Here's how the part is built. I have some questions about the finished solid (model axes, mm). A direction names the side the tool comes from. Round coordinates to 2 decimals unless told otherwise and drop trailing zeros. Loops run counter-clockwise (first coordinate to the right, second up) from the corner with the lowest first, then second, coordinate; pieces in that order, holes last. Notation, with made-up numbers: (52.5, 60) -> (57.5, 60) arc R16 cw to (57.5, 87) -> close; hole circle Ø6 at (-32.75, -33.5). An arc over 180 degrees is marked (long way). Use one line per item in the form item = value. Start each with the question number.
Item 1: Thinking about a two-plate mould opening in Z: for faces 1 (the face through (0.15, 207.27, 2.14)), 2 (the face through (-2, 156, 6)), 3 (the face through (2, 119, 4.3)), which applies, released by +Z, released by -Z, zero draft, split by the parting line, or undercut?
Item 2: If we section it at A-A (y = 172): Write out the boundary of the cut face in (x, z) (3 decimals).
Item 3: For faces 4 (the face through (-1.57, 205.91, 3.09)), 5 (the face through (-2, 21, 6)), 6 (the face through (-3, 238, 4)), which set-ups out of +Z, -Z, +X, -X, +Y, -Y let a thin tool reach every point of the face, with its end or its side?
Item 4: I'm going to push flat-ended pins straight in: pin 1 Ø3 at (y, z) = (20, 4.914) entering from -X; pin 2 Ø4 at (y, z) = (20.5, 4) entering from -X; pin 3 Ø0.6 at (x, y) = (1, 31) entering from +Z; pin 4 Ø2 at (y, z) = (85, 4.914) entering from +X. Where does each tip first touch, or does it pass through?
Item 5: If I drill on L1, parallel to Z at x = -1.25, y = 20; L2, parallel to Y at x = -4.25, z = 3.5; L3, parallel to Y at x = 1, z = 2, over which ranges is the centre line in solid material (lowest first)? Write a range as [from, to].
Autodesk Fusion 360 part; units mm, degrees
sketch "Skizze1" plane through (0, 0, 0) normal (0, 1, 0) x (1, 0, 0)
  line L0 (-29.0267, 0) -> (32.308, 0) construction
  line L1 (0, -25.3668) -> (0, 26.124) construction
  line L2 (0, 0) -> (0, -10)
  line L3 (0, -10) -> (-3, -10)
  line L4 (0, 0) -> (-6.815, 0)
  line L5 (-3, -10) -> (-6.815, 0)
  dimension "d1" = 10
  dimension "d2" = 6.815
  dimension "d3" = 3
extrude "Extrusion1" add sketch "Skizze1" along normal blind 238
sketch "Skizze2" plane through (0, 0, 0) normal (1, 0, 0) x (0, 1, 0)
  line L0 (0, 32.3505) -> (0, -25.958) construction
  line L1 (-11.6611, 0) -> (310, 0) construction
  line L2 (119, 63.4137) -> (119, -57.7153) construction
  line L3 (20, 43.9775) -> (20, -44.5265) construction
  line L4 (220, 51.6132) -> (220, -50) construction
  line L5 (85, 33.2182) -> (85, -47.6502) construction
  line L6 (155, 33.2182) -> (155, -42.444) construction
  line L7 (261.5293, 4.914) -> (-37.3941, 4.914) construction
  circle A0 centre (220, 4.914) radius 1.25
  circle A1 centre (220, 4.914) radius 2.5
  circle A2 centre (155, 4.914) radius 1.25
  circle A3 centre (155, 4.914) radius 2.5
  circle A4 centre (85, 4.914) radius 1.25
  circle A5 centre (85, 4.914) radius 2.5
  circle A6 centre (20, 4.914) radius 1.25
  circle A7 centre (20, 4.914) radius 2.5
  line L8 (207, 25.1754) -> (207, -27.1787) construction
  line L9 (32, 29.9975) -> (32, -45.4338) construction
  line L10 (257.1127, 6.878) -> (-52.1736, 6.878) construction
  line L11 (203.5, 0) -> (210.5, 0)
  line L12 (210.5, 0) -> (210.5, 6.878)
  line L13 (210.5, 6.878) -> (203.5, 6.878)
  line L14 (203.5, 6.878) -> (203.5, 0)
  line L15 (203.5, 0) -> (210.5, 6.878) construction
  line L16 (210.5, 0) -> (203.5, 6.878) construction
  line L17 (115.5, 0) -> (122.5, 0)
  line L18 (122.5, 0) -> (122.5, 6.878)
  line L19 (122.5, 6.878) -> (115.5, 6.878)
  line L20 (115.5, 6.878) -> (115.5, 0)
  line L21 (115.5, 0) -> (122.5, 6.878) construction
  line L22 (122.5, 0) -> (115.5, 6.878) construction
  line L23 (28.5, 0) -> (35.5, 0)
  line L24 (35.5, 0) -> (35.5, 6.878)
  line L25 (35.5, 6.878) -> (28.5, 6.878)
  line L26 (28.5, 6.878) -> (28.5, 0)
  line L27 (28.5, 0) -> (35.5, 6.878) construction
  line L28 (35.5, 0) -> (28.5, 6.878) construction
  point P0 (207, 3.439)
  point P1 (119, 3.439)
  point P2 (32, 3.439)
  dimension "d6" = 119
  dimension "d7" = 101
  dimension "d8" = 99
  dimension "d9" = 34
  dimension "d10" = 36
  dimension "d11" = 4.914
  dimension "d12" = 2.5
  dimension "d13" = 5
  dimension "d14" = 2.5
  dimension "d15" = 5
  dimension "d16" = 2.5
  dimension "d17" = 5
  dimension "d18" = 2.5
  dimension "d19" = 5
  dimension "d24" = 87
  dimension "d25" = 88
  dimension "d26" = 6.878
  dimension "d27" = 7
  dimension "d28" = 7
  dimension "d29" = 7
extrude "Extrusion2" cut sketch "Skizze2" against normal blind 10 contours A0 | A1 | A2 | A3 | A4 | A5 | A6 | A7
extrude "Extrusion3" add sketch "Skizze2" against normal blind 2 contours A1 | A3 | A5 | A7
extrude "Extrusion4" add sketch "Skizze2" along normal blind 2 contours L11 L12 L13 L14 | L17 L18 L19 L20 | L23 L24 L25 L26
sketch "Skizze3" plane through (-5.9491, 0, 2.2696) normal (-0.9343, 0, 0.3564) x (0, -1, 0)
  ellipse E0 centre (-155, 2.8303) end of major axis (-155, 0.1546) minor radius 2.5
  ellipse E1 centre (-85, 2.8303) end of major axis (-85, 0.1546) minor radius 2.5
  ellipse E2 centre (-220, 2.8303) end of major axis (-220, 0.1546) minor radius 2.5
  ellipse E3 centre (-20, 2.8303) end of major axis (-20, 0.1546) minor radius 2.5
  line L0 (0, -2.4292) -> (0, 8.2738)
  line L1 (0, 8.2738) -> (-238, 8.2738)
  line L2 (-238, 8.2738) -> (-238, -2.4292)
  line L3 (-238, -2.4292) -> (0, -2.4292)
  line L4 (-256.1946, 8.2738) -> (13.3488, 8.2738) construction
  line L5 (-271.6873, 3.2738) -> (21.7349, 3.2738) construction
  line L6 (0, 76.206) -> (0, -63.9663) construction
  line L7 (-207, 69.0398) -> (-207, -61.5402) construction
  line L8 (-119, 70) -> (-119, -67.3252) construction
  line L9 (-32, 63.2186) -> (-32, -40) construction
  circle A0 centre (-207, 3.2738) radius 1.25
  circle A1 centre (-119, 3.2738) radius 1.25
  circle A2 centre (-32, 3.2738) radius 1.25
  line L10 (-205.7298, 1.0738) -> (-204.4597, 3.2738)
  line L11 (-204.4597, 3.2738) -> (-205.7298, 5.4738)
  line L12 (-205.7298, 5.4738) -> (-208.2702, 5.4738)
  line L13 (-208.2702, 5.4738) -> (-209.5403, 3.2738)
  line L14 (-209.5403, 3.2738) -> (-208.2702, 1.0738)
  line L15 (-208.2702, 1.0738) -> (-205.7298, 1.0738)
  line L16 (-117.7298, 1.0738) -> (-116.4597, 3.2738)
  line L17 (-116.4597, 3.2738) -> (-117.7298, 5.4738)
  line L18 (-117.7298, 5.4738) -> (-120.2702, 5.4738)
  line L19 (-120.2702, 5.4738) -> (-121.5403, 3.2738)
  line L20 (-121.5403, 3.2738) -> (-120.2702, 1.0738)
  line L21 (-120.2702, 1.0738) -> (-117.7298, 1.0738)
  line L22 (-30.7298, 1.0738) -> (-29.4597, 3.2738)
  line L23 (-29.4597, 3.2738) -> (-30.7298, 5.4738)
  line L24 (-30.7298, 5.4738) -> (-33.2702, 5.4738)
  line L25 (-33.2702, 5.4738) -> (-34.5403, 3.2738)
  line L26 (-34.5403, 3.2738) -> (-33.2702, 1.0738)
  line L27 (-33.2702, 1.0738) -> (-30.7298, 1.0738)
  point P0 (-207, 3.2738)
  point P1 (-119, 3.2738)
  point P2 (-32, 3.2738)
  dimension "d32" = 5
  dimension "d35" = 119
  dimension "d36" = 87
  dimension "d37" = 88
  dimension "d38" = 2.5
  dimension "d39" = 2.5
  dimension "d40" = 2.5
  dimension "d41" = 4.4
  dimension "d42" = 4.4
  dimension "d43" = 4.4
extrude "Extrusion5" cut sketch "Skizze3" against normal blind 8 contours A0 | A1 | A2
extrude "Extrusion6" cut sketch "Skizze3" against normal blind 3.8 contours L10 L11 L12 L13 L14 L15 | L16 L17 L18 L19 L20 L21 | L22 L23 L24 L25 L26 L27
extrude "Extrusion7" add sketch "Skizze3" against normal blind 2 contours L10 L11 L12 L13 L14 L15 | L16 L17 L18 L19 L20 L21 | L22 L23 L24 L25 L26 L27
Values found:
q1.face_1 = undercut
q1.face_2 = undercut
q1.face_3 = zero draft
q2.outline = (-6.815, 0) -> (0, 0) -> (0, 10) -> (-3, 10) -> close
q3.face_4 = none
q3.face_5 = -X
q3.face_6 = +Z, -Z, +X, -X, +Y
q4.pin_1 = -2
q4.pin_2 = -6.05
q4.pin_3 = 6.88
q4.pin_4 = through
q5.L1 = [0, 3.66], [6.16, 10]
q5.L2 = [0, 17.94], [22.06, 82.94], [87.06, 152.94], [157.06, 217.94], [222.06, 238]
q5.L3 = [28.5, 31.32], [32.68, 35.5], [115.5, 118.32], [119.68, 122.5], [203.5, 206.32], [207.68, 210.5]
